The model under review builds one solid part; all positions refer to its coordinate system, in mm. Face numbers are marked on the shaded views. A direction names the side the tool comes from. Round coordinates to 2 decimals unless told otherwise and drop trailing zeros. Order: outer loops, then holes, each group sorted by start corner. A loop starts at its lowest first (then second) coordinate and runs counter-clockwise, first axis right, second up. Notation, with made-up numbers: M 36.25,8 L 85.25,8 A10 ccw 85.25,24 Z; hole C 21,40 d7. An arc over 180 degrees is marked long. Answer as a JSON object with one key per item and string values. Group by question number.
1) For the marked faces 3 and 4, list the 3-axis set-ups (+Z, -Z, +X, -X, +Y, -Y) from which the entire face can be reached by the end or side of a thin tool; tool diameter is ignored.
2) Consider section B-B, the plane x = 221. Write out the cut boundary in (y, z), then the cut area to 3 significant figures.
3) To check wall thickness, follow line 1 (Z direction, x = 81, y = 18.5); line 2 (Y direction, x = 123, z = 4.75); line 3 (Z direction, x = 115.5, y = 4.25). State the ranges of each line that lie inside material, in increasing order.
4) Insertion check: pin 1 Ø4 at (x, y) = (197.5, 16.5) entering from -Z; pin 2 Ø4.5 at (x, y) = (239, 12.5) entering from +Z; pin 3 Ø2 at (x, y) = (63, 10) entering from -Z. Each pin has a flat end and moves straight along its axis. Give the tip position at first contact, or say it passes through.
5) Consider section A-A, the plane x = 173. Write out the cut boundary in (y, z).
6) The part is to be moulded in two halves that separate along X. For the marked faces 1 and 2, say which applies: +X half, -X half, draft (parallel to the pull), parting line (faces both ways), or undercut.
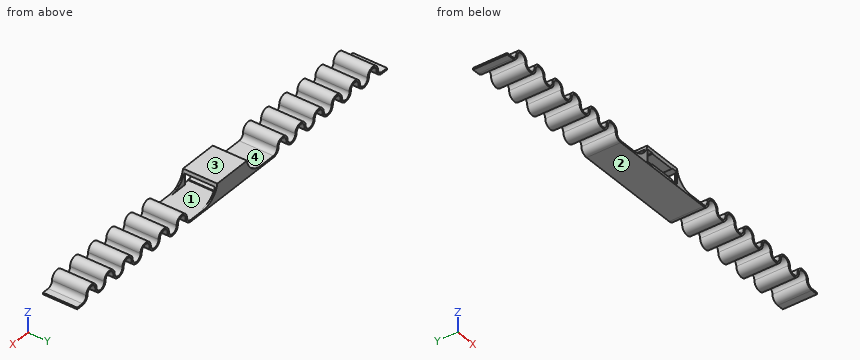
Autodesk Fusion 360 part; units mm, degrees
sketch "Sketch1" plane through (0, 0, 0) normal (0, 0, 1) x (1, 0, 0)
  line L0 (0, 0) -> (240, 0)
  line L1 (240, 0) -> (240, 20)
  line L2 (240, 20) -> (0, 20)
  line L3 (0, 20) -> (0, 0)
  line L4 (120, 0) -> (120, 20) construction
  line L5 (130, 20) -> (110, 20)
  line L6 (110, 20) -> (110, 0)
  line L7 (110, 0) -> (130, 0)
  line L8 (130, 0) -> (130, 20)
  line L9 (130, 20) -> (110, 0) construction
  line L10 (110, 20) -> (130, 0) construction
  line L11 (127.5, 19) -> (112.5, 19)
  line L12 (112.5, 19) -> (112.5, 1)
  line L13 (112.5, 1) -> (127.5, 1)
  line L14 (127.5, 1) -> (127.5, 19)
  line L15 (127.5, 19) -> (112.5, 1) construction
  line L16 (112.5, 19) -> (127.5, 1) construction
  point P0 (120, 10)
  point P1 (120, 10)
  dimension "d1" = 240
  dimension "d2" = 20
  dimension "d3" = 20
  dimension "d4" = 15
  dimension "d5" = 18
extrude "Extrude1" add sketch "Sketch1" along normal blind 10 contours L0 L2 L3 L6 | L0 L2 L5 L6 L7 L8 | L0 L1 L2 L8 | L11 L12 L13 L14
sketch "Sketch2" plane through (0, 0, 0) normal (0, -1, 0) x (1, 0, 0)
  line L0 (0, 0) -> (240, 0)
  line L1 (240, 0) -> (240, 10)
  line L2 (240, 10) -> (0, 10)
  line L3 (0, 10) -> (0, 0)
  line L4 (0, 4) -> (100, 4) construction
  arc A0 (4, 1) -> (7, 4) centre (4, 4) ccw
  arc A1 (4, 0) -> (8, 4) centre (4, 4) ccw
  arc A2 (15, 4) -> (7, 4) centre (11, 4) ccw
  arc A3 (14, 4) -> (8, 4) centre (11, 4) ccw
  arc A4 (14, 4) -> (22, 4) centre (18, 4) ccw
  arc A5 (15, 4) -> (21, 4) centre (18, 4) ccw
  arc A6 (29, 4) -> (21, 4) centre (25, 4) ccw
  arc A7 (28, 4) -> (22, 4) centre (25, 4) ccw
  arc A8 (28, 4) -> (36, 4) centre (32, 4) ccw
  arc A9 (29, 4) -> (35, 4) centre (32, 4) ccw
  arc A10 (43, 4) -> (35, 4) centre (39, 4) ccw
  arc A11 (42, 4) -> (36, 4) centre (39, 4) ccw
  arc A12 (42, 4) -> (50, 4) centre (46, 4) ccw
  arc A13 (43, 4) -> (49, 4) centre (46, 4) ccw
  arc A14 (57, 4) -> (49, 4) centre (53, 4) ccw
  arc A15 (56, 4) -> (50, 4) centre (53, 4) ccw
  arc A16 (56, 4) -> (64, 4) centre (60, 4) ccw
  arc A17 (57, 4) -> (63, 4) centre (60, 4) ccw
  arc A18 (71, 4) -> (63, 4) centre (67, 4) ccw
  arc A19 (70, 4) -> (64, 4) centre (67, 4) ccw
  arc A20 (70, 4) -> (78, 4) centre (74, 4) ccw
  arc A21 (71, 4) -> (77, 4) centre (74, 4) ccw
  arc A22 (85, 4) -> (77, 4) centre (81, 4) ccw
  arc A23 (84, 4) -> (78, 4) centre (81, 4) ccw
  line L5 (0, 0) -> (0, 1) construction
  line L6 (0, 1) -> (98.101, 1) construction
  line L7 (98.101, 1) -> (88, 1)
  arc A24 (85, 4) -> (88, 1) centre (88, 4) ccw
  arc A25 (84, 4) -> (88, 0) centre (88, 4) ccw
  line L8 (4, 1) -> (0, 1)
  line L9 (4, 0) -> (0, 0)
  line L10 (98.101, 1) -> (98.101, 0)
  line L11 (120, 10) -> (120, 0) construction
  line L12 (131.5, 10) -> (108.5, 10)
  line L13 (108.5, 10) -> (108.5, 0)
  line L14 (108.5, 0) -> (131.5, 0)
  line L15 (131.5, 0) -> (131.5, 10)
  line L16 (131.5, 10) -> (108.5, 0) construction
  line L17 (108.5, 10) -> (131.5, 0) construction
  arc A26 (98.101, 1) -> (108.5, 10) centre (98.101, 11.5078) ccw
  point P0 (120, 5)
  dimension "d53" = 4
  dimension "d55" = 8
  dimension "d56" = 6
  dimension "d57" = 8
  dimension "d58" = 6
  dimension "d65" = 1
  dimension "d66" = 8
  dimension "d67" = 6
  dimension "d73" = 23
extrude "Extrude2" cut sketch "Sketch2" against normal blind 30 contours L0 A1 A3 A4 | L2 L3 A0 A2 A5 A6 A9 A10 A13 A14 A17 A18 A21 A22 L7 A24 L8 A26 | L0 A4 A7 A8 | L0 A8 A11 A12 | L0 A12 A15 A16 | L0 A16 A19 A20 | L0 A20 A23 A25
ref_plane "WorkPlane1" through (120, 0, 0) normal (1, 0, 0) x (0, 1, 0)
mirror "Mirror1" about plane through (120, 0, 0) normal (1, 0, 0) of "Extrude2"
sketch "Sketch3" plane through (0, 0, 0) normal (0, -1, 0) x (1, 0, 0)
  arc A0 (152, 0) -> (156, 4) centre (152, 4) ccw
  arc A1 (162, 4) -> (156, 4) centre (159, 4) ccw
  arc A2 (162, 4) -> (170, 4) centre (166, 4) ccw
  arc A3 (176, 4) -> (170, 4) centre (173, 4) ccw
  arc A4 (176, 4) -> (184, 4) centre (180, 4) ccw
  arc A5 (190, 4) -> (184, 4) centre (187, 4) ccw
  arc A6 (190, 4) -> (198, 4) centre (194, 4) ccw
  arc A7 (204, 4) -> (198, 4) centre (201, 4) ccw
  arc A8 (204, 4) -> (212, 4) centre (208, 4) ccw
  arc A9 (218, 4) -> (212, 4) centre (215, 4) ccw
  arc A10 (218, 4) -> (226, 4) centre (222, 4) ccw
  arc A11 (232, 4) -> (226, 4) centre (229, 4) ccw
  arc A12 (232, 4) -> (236, 0) centre (236, 4) ccw
  line L0 (236, 0) -> (240, 0)
  line L1 (240, 0) -> (240, 1)
  line L2 (240, 1) -> (236, 1)
  arc A13 (233, 4) -> (236, 1) centre (236, 4) ccw
  arc A14 (233, 4) -> (225, 4) centre (229, 4) ccw
  arc A15 (219, 4) -> (225, 4) centre (222, 4) ccw
  arc A16 (219, 4) -> (211, 4) centre (215, 4) ccw
  arc A17 (205, 4) -> (211, 4) centre (208, 4) ccw
  arc A18 (205, 4) -> (197, 4) centre (201, 4) ccw
  arc A19 (191, 4) -> (197, 4) centre (194, 4) ccw
  arc A20 (191, 4) -> (183, 4) centre (187, 4) ccw
  arc A21 (177, 4) -> (183, 4) centre (180, 4) ccw
  arc A22 (177, 4) -> (169, 4) centre (173, 4) ccw
  arc A23 (163, 4) -> (169, 4) centre (166, 4) ccw
  arc A24 (163, 4) -> (155, 4) centre (159, 4) ccw
  arc A25 (152, 1) -> (155, 4) centre (152, 4) ccw
  line L3 (152, 1) -> (141.899, 1)
  line L4 (131.5, 10) -> (108.5, 10)
  line L5 (98.101, 1) -> (88, 1)
  arc A26 (85, 4) -> (88, 1) centre (88, 4) ccw
  arc A27 (85, 4) -> (77, 4) centre (81, 4) ccw
  arc A28 (71, 4) -> (77, 4) centre (74, 4) ccw
  arc A29 (71, 4) -> (63, 4) centre (67, 4) ccw
  arc A30 (57, 4) -> (63, 4) centre (60, 4) ccw
  arc A31 (57, 4) -> (49, 4) centre (53, 4) ccw
  arc A32 (43, 4) -> (49, 4) centre (46, 4) ccw
  arc A33 (43, 4) -> (35, 4) centre (39, 4) ccw
  arc A34 (29, 4) -> (35, 4) centre (32, 4) ccw
  arc A35 (29, 4) -> (21, 4) centre (25, 4) ccw
  arc A36 (15, 4) -> (21, 4) centre (18, 4) ccw
  arc A37 (15, 4) -> (7, 4) centre (11, 4) ccw
  arc A38 (4, 1) -> (7, 4) centre (4, 4) ccw
  line L6 (4, 1) -> (0, 1)
  line L7 (0, 1) -> (0, 0)
  line L8 (0, 0) -> (4, 0)
  arc A39 (4, 0) -> (8, 4) centre (4, 4) ccw
  arc A40 (14, 4) -> (8, 4) centre (11, 4) ccw
  arc A41 (14, 4) -> (22, 4) centre (18, 4) ccw
  arc A42 (28, 4) -> (22, 4) centre (25, 4) ccw
  arc A43 (28, 4) -> (36, 4) centre (32, 4) ccw
  arc A44 (42, 4) -> (36, 4) centre (39, 4) ccw
  arc A45 (42, 4) -> (50, 4) centre (46, 4) ccw
  arc A46 (56, 4) -> (50, 4) centre (53, 4) ccw
  arc A47 (56, 4) -> (64, 4) centre (60, 4) ccw
  arc A48 (70, 4) -> (64, 4) centre (67, 4) ccw
  arc A49 (70, 4) -> (78, 4) centre (74, 4) ccw
  arc A50 (84, 4) -> (78, 4) centre (81, 4) ccw
  arc A51 (84, 4) -> (88, 0) centre (88, 4) ccw
  line L9 (88, 0) -> (152, 0)
  arc A52 (131.5, 10) -> (141.899, 1) centre (141.899, 11.5078) ccw
  arc A53 (98.101, 1) -> (108.5, 10) centre (98.101, 11.5078) ccw
sketch "Sketch4" plane through (0, 0, 0) normal (0, -1, 0) x (1, 0, 0)
  line L0 (108.5, 10) -> (131.5, 10) construction
  line L1 (131.5, 10) -> (131.5, 0) construction
  line L2 (131.5, 0) -> (108.5, 0) construction
  line L3 (108.5, 0) -> (108.5, 10) construction
  line L4 (88, 0) -> (152, 0)
  line L5 (108.5, 0) -> (131.5, 0) construction
  line L6 (131.5, 0) -> (131.5, 1) construction
  line L7 (131.5, 1) -> (108.5, 1) construction
  line L8 (108.5, 1) -> (108.5, 0) construction
  line L9 (108.5, 1) -> (131.5, 1) construction
  line L10 (131.5, 1) -> (131.5, 1.5) construction
  line L11 (131.5, 1.5) -> (108.5, 1.5)
  line L12 (108.5, 1.5) -> (108.5, 1) construction
  line L13 (131.5, 1.5) -> (108.5, 1.5)
  line L14 (108.5, 1.5) -> (108.5, 7.5)
  line L15 (108.5, 7.5) -> (131.5, 7.5)
  line L16 (131.5, 7.5) -> (131.5, 1.5)
  line L17 (127.5006, 1) -> (112.5006, 1)
  line L18 (112.5006, 1) -> (112.5006, 1.5)
  line L19 (127.5006, 1.5) -> (127.5006, 1)
  line L20 (127.5006, 1) -> (120, 1.5) construction
  line L21 (112.5006, 1) -> (120, 1.5) construction
  line L22 (112.5, 7.5) -> (112.5, 8)
  line L23 (112.5, 8) -> (127.5, 8)
  line L24 (127.5, 8) -> (127.5, 7.5)
  line L25 (120, 7.5) -> (112.5, 8) construction
  line L26 (120, 7.5) -> (127.5, 8) construction
  line L27 (127.5, 7.5) -> (127.5, 1.5) construction
  line L28 (127.5, 8) -> (131.5, 8)
  line L29 (131.5, 8) -> (131.5, 7.5)
  line L30 (112.5, 8) -> (108.5, 8)
  line L31 (108.5, 8) -> (108.5, 7.5)
  line L32 (108.5, 1.5) -> (108.5, 1)
  line L33 (112.5006, 1) -> (108.5, 1)
  line L34 (131.5, 1.5) -> (131.5, 1)
  line L35 (131.5, 1) -> (127.5006, 1)
  point P0 (108.5, 10)
  dimension "d74" = 1
  dimension "d75" = 0.5
  dimension "d76" = 6
  dimension "d78" = 15
  dimension "d80" = 0.5
  dimension "d81" = 15
extrude "Extrude3" cut sketch "Sketch4" against normal blind 19 contours L11 L13 L19 L34 L35 | L11 L13 L14 L15 L16 | L15 L24 L28 L29 | L11 L13 L18 L32 L33 | L15 L22 L30 L31
sketch "Sketch5" plane through (108.5, 0, 0) normal (1, 0, 0) x (0, 1, 0)
  line L0 (0, 8) -> (0, 1)
  line L1 (0, 1) -> (19, 1)
  line L2 (19, 1) -> (19, 8)
  line L3 (19, 8) -> (0, 8)
  line L4 (19, 8) -> (1, 8)
  line L5 (1, 8) -> (1, 1)
  line L6 (1, 1) -> (19, 1)
  line L7 (19, 1) -> (19, 8)
  dimension "d84" = 18
extrude "Extrude4" cut sketch "Sketch5" against normal blind 12 contours L1 L2 L3 L4 L5 L6 L7
sketch "Sketch6" plane through (131.5, 0, 0) normal (-1, 0, 0) x (0, -1, 0)
  line L0 (0, 1) -> (0, 8)
  line L1 (0, 8) -> (-19, 8)
  line L2 (-19, 8) -> (-19, 1)
  line L3 (-19, 1) -> (0, 1)
  line L4 (-19, 1) -> (-1, 1)
  line L5 (-1, 1) -> (-1, 8)
  line L6 (-1, 8) -> (-19, 8)
  line L7 (-19, 8) -> (-19, 1)
  dimension "d87" = 18
extrude "Extrude5" cut sketch "Sketch6" against normal blind 11 contours L1 L2 L3 L4 L5 L6 L7
sketch "Sketch7" plane through (0, 0, 0) normal (0, -1, 0) x (1, 0, 0)
  line L0 (112.5, 7.5) -> (127.5, 7.5)
  line L1 (127.5, 7.5) -> (127.5, 8)
  line L2 (127.5, 8) -> (131.5, 8)
  line L3 (131.5, 8) -> (131.5, 1)
  line L4 (131.5, 1) -> (127.5006, 1)
  line L5 (127.5006, 1) -> (127.5006, 1.5)
  line L6 (127.5006, 1.5) -> (112.5006, 1.5)
  line L7 (112.5006, 1.5) -> (112.5006, 1)
  line L8 (112.5006, 1) -> (108.5, 1)
  line L9 (108.5, 1) -> (108.5, 8)
  line L10 (108.5, 8) -> (112.5, 8)
  line L11 (112.5, 8) -> (112.5, 7.5)
  arc A0 (152, 0) -> (156, 4) centre (152, 4) ccw
  arc A1 (162, 4) -> (156, 4) centre (159, 4) ccw
  arc A2 (162, 4) -> (170, 4) centre (166, 4) ccw
  arc A3 (176, 4) -> (170, 4) centre (173, 4) ccw
  arc A4 (176, 4) -> (184, 4) centre (180, 4) ccw
  arc A5 (190, 4) -> (184, 4) centre (187, 4) ccw
  arc A6 (190, 4) -> (198, 4) centre (194, 4) ccw
  arc A7 (204, 4) -> (198, 4) centre (201, 4) ccw
  arc A8 (204, 4) -> (212, 4) centre (208, 4) ccw
  arc A9 (218, 4) -> (212, 4) centre (215, 4) ccw
  arc A10 (218, 4) -> (226, 4) centre (222, 4) ccw
  arc A11 (232, 4) -> (226, 4) centre (229, 4) ccw
  arc A12 (232, 4) -> (236, 0) centre (236, 4) ccw
  line L12 (236, 0) -> (240, 0)
  line L13 (240, 0) -> (240, 1)
  line L14 (240, 1) -> (236, 1)
  arc A13 (233, 4) -> (236, 1) centre (236, 4) ccw
  arc A14 (233, 4) -> (225, 4) centre (229, 4) ccw
  arc A15 (219, 4) -> (225, 4) centre (222, 4) ccw
  arc A16 (219, 4) -> (211, 4) centre (215, 4) ccw
  arc A17 (205, 4) -> (211, 4) centre (208, 4) ccw
  arc A18 (205, 4) -> (197, 4) centre (201, 4) ccw
  arc A19 (191, 4) -> (197, 4) centre (194, 4) ccw
  arc A20 (191, 4) -> (183, 4) centre (187, 4) ccw
  arc A21 (177, 4) -> (183, 4) centre (180, 4) ccw
  arc A22 (177, 4) -> (169, 4) centre (173, 4) ccw
  arc A23 (163, 4) -> (169, 4) centre (166, 4) ccw
  arc A24 (163, 4) -> (155, 4) centre (159, 4) ccw
  arc A25 (152, 1) -> (155, 4) centre (152, 4) ccw
  line L15 (152, 1) -> (141.899, 1)
  arc A26 (131.5, 10) -> (141.899, 1) centre (141.899, 11.5078) ccw
  line L16 (131.5, 10) -> (108.5, 10)
  arc A27 (98.101, 1) -> (108.5, 10) centre (98.101, 11.5078) ccw
  line L17 (98.101, 1) -> (88, 1)
  arc A28 (85, 4) -> (88, 1) centre (88, 4) ccw
  arc A29 (85, 4) -> (77, 4) centre (81, 4) ccw
  arc A30 (71, 4) -> (77, 4) centre (74, 4) ccw
  arc A31 (71, 4) -> (63, 4) centre (67, 4) ccw
  arc A32 (57, 4) -> (63, 4) centre (60, 4) ccw
  arc A33 (57, 4) -> (49, 4) centre (53, 4) ccw
  arc A34 (43, 4) -> (49, 4) centre (46, 4) ccw
  arc A35 (43, 4) -> (35, 4) centre (39, 4) ccw
  arc A36 (29, 4) -> (35, 4) centre (32, 4) ccw
  arc A37 (29, 4) -> (21, 4) centre (25, 4) ccw
  arc A38 (15, 4) -> (21, 4) centre (18, 4) ccw
  arc A39 (15, 4) -> (7, 4) centre (11, 4) ccw
  arc A40 (4, 1) -> (7, 4) centre (4, 4) ccw
  line L18 (4, 1) -> (0, 1)
  line L19 (0, 1) -> (0, 0)
  line L20 (0, 0) -> (4, 0)
  arc A41 (4, 0) -> (8, 4) centre (4, 4) ccw
  arc A42 (14, 4) -> (8, 4) centre (11, 4) ccw
  arc A43 (14, 4) -> (22, 4) centre (18, 4) ccw
  arc A44 (28, 4) -> (22, 4) centre (25, 4) ccw
  arc A45 (28, 4) -> (36, 4) centre (32, 4) ccw
  arc A46 (42, 4) -> (36, 4) centre (39, 4) ccw
  arc A47 (42, 4) -> (50, 4) centre (46, 4) ccw
  arc A48 (56, 4) -> (50, 4) centre (53, 4) ccw
  arc A49 (56, 4) -> (64, 4) centre (60, 4) ccw
  arc A50 (70, 4) -> (64, 4) centre (67, 4) ccw
  arc A51 (70, 4) -> (78, 4) centre (74, 4) ccw
  arc A52 (84, 4) -> (78, 4) centre (81, 4) ccw
  arc A53 (84, 4) -> (88, 0) centre (88, 4) ccw
  line L21 (88, 0) -> (152, 0)
equation "d57 = d55"
equation "d58 = d56"
equation "d66 = d55"
equation "d67 = d56"
Results list:
{
 "1": {"face 3": "+Z, +X, -X, +Y, -Y", "face 4": "none"},
 "2": {"outline": "M 0,0.13 L 20,0.13 L 20,1.17 L 0,1.17 Z", "area": "20.9 mm^2"},
 "3": {"line 1": "7 to 8", "line 2": "19 to 20", "line 3": "0 to 1.5, 7.5 to 10"},
 "4": {"pin 1": "z = 0.29", "pin 2": "z = 1", "pin 3": "z = 0.54"},
 "5": {"outline": "M 0,7 L 20,7 L 20,8 L 0,8 Z"},
 "6": {"face 1": "undercut", "face 2": "draft"}
}
